from build123d import *

# Parameters (mm, degrees)
SKETCH1_W                = 40
SKETCH1_H                = 30
BOSS_EXTRUDE1_DEPTH      = 15
SKETCH2_W                = 99.5
SKETCH2_H                = 60
BOSS_EXTRUDE2_DEPTH      = 10
M3_CLEARANCE_HOLE1_D     = 3.2
SKETCH7_W                = 105.85
SKETCH7_H                = 66.35
SKETCH7_W_2              = 99.5
SKETCH7_H_2              = 60
BOSS_EXTRUDE3_DEPTH      = 3
CUT_EXTRUDE2_DEPTH       = 1.25
M3_CLEARANCE_HOLE3_D     = 3.2
M3_CLEARANCE_HOLE3_DEPTH = 12
M3_CLEARANCE_HOLE3_TIP   = 0.96137699
F_1_4_CLEARANCE_HOLE3_D  = 6.5278
SKETCH20_R               = 2.8
SKETCH20_R_2             = 5
CUT_EXTRUDE4_DEPTH       = 21
SKETCH23_W               = 6.48
SKETCH23_H               = 3
BOSS_EXTRUDE5_DEPTH      = 10
SKETCH43_W               = 6
SKETCH43_H               = 3
BOSS_EXTRUDE7_DEPTH      = 18
F_1_4_CLEARANCE_HOLE2_D  = 6.5278
CUT_EXTRUDE9_START       = -22
CUT_EXTRUDE9_DEPTH       = 22
SKETCH45_W               = 45
SKETCH45_H               = 60
CUT_EXTRUDE10_DEPTH      = 5
CUT_EXTRUDE11_DEPTH      = 1.25
M3_CLEARANCE_HOLE5_D     = 3.2
M3_CLEARANCE_HOLE5_DEPTH = 10
M3_CLEARANCE_HOLE5_TIP   = 0.96137699
FILLET3_R                = 2
FILLET4_R                = 1


with BuildPart() as part:
    # Sketch1 → Boss-Extrude1 (new body)
    with BuildSketch(Plane(origin=(0, 0, 0), x_dir=(1, 0, 0), z_dir=(0, 1, 0))):
        Rectangle(SKETCH1_W, SKETCH1_H)
    extrude(amount=-BOSS_EXTRUDE1_DEPTH)

    # Sketch2 → Boss-Extrude2 (add)
    with BuildSketch(Plane.XZ.offset(15)):
        with Locations((25.25, 0)):
            Rectangle(SKETCH2_W, SKETCH2_H)
    extrude(amount=BOSS_EXTRUDE2_DEPTH)

    # M3 Clearance Hole1 (through all)
    with Locations(Plane(origin=(0, 0, 0), x_dir=(1, 0, 0), z_dir=(0, 1, 0))):
        with Locations((-16.5, 11.5), (16.5, 11.5), (-16.5, -11.5), (16.5, -11.5)):
            Hole(M3_CLEARANCE_HOLE1_D / 2)

    # Sketch7 → Boss-Extrude3 (add)
    with BuildSketch(Plane.XZ.offset(25)):
        with Locations((25.25, 0)):
            Rectangle(SKETCH7_W, SKETCH7_H)
        with Locations((25.25, 0)):
            Rectangle(SKETCH7_W_2, SKETCH7_H_2, mode=Mode.SUBTRACT)
    extrude(amount=-BOSS_EXTRUDE3_DEPTH)

    # Sketch14 → Cut-Extrude2 (cut, symmetric)
    with BuildSketch(Plane.ZY.offset(20.5)):
        Polygon((-27.75, -16.91228676), (-27.75, -15), (-22.25, -15), (-22.25, -16.91228676), (-22.25, -20.08771324), (-25, -21.675426481), (-27.75, -20.08771324), align=None)
        Polygon((22.25, -16.91228676), (22.25, -20.08771324), (25, -21.675426481), (27.75, -20.08771324), (27.75, -16.91228676), (27.75, -15), (22.25, -15), align=None)
    extrude(amount=CUT_EXTRUDE2_DEPTH, both=True, mode=Mode.SUBTRACT)

    # M3 Clearance Hole3
    with Locations(Plane.ZY.offset(24.5)):
        with Locations((-25, -18.5), (25, -18.5)):
            Hole(M3_CLEARANCE_HOLE3_D / 2, depth=M3_CLEARANCE_HOLE3_DEPTH)
            with Locations((0, 0, -(M3_CLEARANCE_HOLE3_DEPTH + M3_CLEARANCE_HOLE3_TIP / 2))):  # 118° drill point
                Cone(0, M3_CLEARANCE_HOLE3_D / 2, M3_CLEARANCE_HOLE3_TIP, mode=Mode.SUBTRACT)

    # 1/4 Clearance Hole3 (through all)
    with Locations(Plane(origin=(0, 0, 0), x_dir=(1, 0, 0), z_dir=(0, 1, 0))):
        with Locations((-12, 0)):
            Hole(F_1_4_CLEARANCE_HOLE3_D / 2)

    # Sketch20 → Cut-Extrude4 (cut)
    with BuildSketch(Plane.XZ.offset(25)):
        with Locations(Location((-16.5, 11.5, 0), (0, 0, 270))):
            Circle(SKETCH20_R)
        with Locations(Location((16.5, 11.5, 0), (0, 0, 270))):
            Circle(SKETCH20_R)
        with Locations(Location((16.5, -11.5, 0), (0, 0, 270))):
            Circle(SKETCH20_R)
        with Locations(Location((-16.5, -11.5, 0), (0, 0, 270))):
            Circle(SKETCH20_R)
        with Locations(Location((-12, 0, 0), (0, 0, 270))):
            Circle(SKETCH20_R_2)
    extrude(amount=-CUT_EXTRUDE4_DEPTH, mode=Mode.SUBTRACT)

    # Sketch23 → Boss-Extrude5 (add, symmetric)
    with BuildSketch(Plane.XY):
        with Locations((0, -26.5)):
            Rectangle(SKETCH23_W, SKETCH23_H)
    extrude(amount=BOSS_EXTRUDE5_DEPTH, both=True)

    # Sketch43 → Boss-Extrude7 (add)
    with BuildSketch(Plane(origin=(0, -15, 0), x_dir=(1, 0, 0), z_dir=(0, 1, 0))):
        with Locations((-13, 16.5)):
            Rectangle(SKETCH43_W, SKETCH43_H)
        with Locations((-13, -16.5)):
            Rectangle(SKETCH43_W, SKETCH43_H)
        with Locations((13, 16.5)):
            Rectangle(SKETCH43_W, SKETCH43_H)
        with Locations((13, -16.5)):
            Rectangle(SKETCH43_W, SKETCH43_H)
    extrude(amount=BOSS_EXTRUDE7_DEPTH)

    # 1/4 Clearance Hole2 (through all)
    with Locations(Plane(origin=(0, -15, 0), x_dir=(1, 0, 0), z_dir=(0, 1, 0))):
        with Locations((0, 22.5), (0, -22.5)):
            Hole(F_1_4_CLEARANCE_HOLE2_D / 2)

    # Sketch44 → Cut-Extrude9 (cut)
    with BuildSketch(Plane(origin=(0, 0, 0), x_dir=(1, 0, 0), z_dir=(0, 1, 0)).offset(CUT_EXTRUDE9_START)):
        Polygon((-6, 15), (6, 15), (6, 7.5), (20, 7.5), (20, -7.5), (6, -7.5), (6, -15), (-6, -15), align=None)
    extrude(amount=CUT_EXTRUDE9_DEPTH, mode=Mode.SUBTRACT)

    # Sketch45 → Cut-Extrude10 (cut)
    with BuildSketch(Plane(origin=(0, -15, 0), x_dir=(1, 0, 0), z_dir=(0, 1, 0))):
        with Locations((42.5, 0)):
            Rectangle(SKETCH45_W, SKETCH45_H)
    extrude(amount=-CUT_EXTRUDE10_DEPTH, mode=Mode.SUBTRACT)

    # Sketch46 → Cut-Extrude11 (cut, symmetric)
    with BuildSketch(Plane(origin=(71, 0, 0), x_dir=(0, 0, -1), z_dir=(1, 0, 0))):
        Polygon((-2.75, -16.91228676), (-2.75, -15), (2.75, -15), (2.75, -16.91228676), (2.75, -20.08771324), (0, -21.675426481), (-2.75, -20.08771324), align=None)
    extrude(amount=CUT_EXTRUDE11_DEPTH, both=True, mode=Mode.SUBTRACT)

    # M3 Clearance Hole5
    with Locations(Plane(origin=(75, 0, 0), x_dir=(0, 0, -1), z_dir=(1, 0, 0))):
        with Locations((0, -18.5)):
            Hole(M3_CLEARANCE_HOLE5_D / 2, depth=M3_CLEARANCE_HOLE5_DEPTH)
            with Locations((0, 0, -(M3_CLEARANCE_HOLE5_DEPTH + M3_CLEARANCE_HOLE5_TIP / 2))):  # 118° drill point
                Cone(0, M3_CLEARANCE_HOLE5_D / 2, M3_CLEARANCE_HOLE5_TIP, mode=Mode.SUBTRACT)

    # Fillet3
    fillet3_edges = [part.edges().sort_by_distance(p)[0] for p in [
        (-10, -6, -18),
        (-16, -6, -18),
        (-10, -6, 18),
        (-16, -6, 18),
        (10, -6, 18),
        (16, -6, 18),
        (10, -6, -18),
        (16, -6, -18),
        (6, -7.5, 15),
        (6, -11, 7.5),
        (20, -10, 7.5),
        (20, -10, -7.5),
        (6, -11, -7.5),
        (6, -7.5, -15),
        (-6, -7.5, -15),
        (-6, -7.5, 15),
        (20, -17.5, 30),
        (65, -17.5, 30),
        (65, -17.5, -30),
        (20, -17.5, -30),
        (-24.5, -18.5, 30),
        (75, -18.5, 30),
        (75, -18.5, -30),
        (-24.5, -18.5, -30),
        (20, -7.5, 15),
        (-20, -7.5, 15),
        (-20, -7.5, -15),
        (20, -7.5, -15),
    ]]
    fillet(fillet3_edges, radius=FILLET3_R)

    # Fillet4
    fillet4_edges = [part.edges().sort_by_distance(p)[0] for p in [
        (-27.675, -23.5, 33.175),
        (78.175, -23.5, 33.175),
        (78.175, -23.5, -33.175),
        (-27.675, -23.5, -33.175),
    ]]
    fillet(fillet4_edges, radius=FILLET4_R)


solid = part.part
Design review of the part built by this model. Coordinates are the model's own, in mm. A direction names the side the tool comes from. Give positions to 0.01 mm unless a question says otherwise; leave off trailing zeros. Loops run counter-clockwise (first coordinate to the right, second up) from the corner with the lowest first, then second, coordinate; pieces in that order, holes last. Notation, with made-up numbers: (32, 11) - (41, 11) arc R33 cw to (41, 50) - close; hole circle Ø9 at (86, 34.5). An arc over 180 degrees is marked (long way). Use CSV: the item, a comma, the result in double quotes. Start each with the question number.
1. Add section A-A (z = -11.5). Count the separate pieces of the cut face and the enclosed holes in it, plus the area to 3 significant figures.
2. Add section C-C (x = 28.5). State the section outline as (y, z) points (3 decimals).
3. Wall thickness on L1, parallel to X at y = -8.5, z = 11.5; L2, parallel to Z at x = -16.5, y = -1.7; L3, parallel to X at y = -2.35, z = -11.5: over which ranges is each line inside the solid? List them lowest first.
4. Draft analysis for pull direction Y (two halves, no side actions). For faces 1 (the flat face through (-20.482, -20.87, -23.606)), 2 (the flat face through (-20, -7, 0)), 3 (the conical face through (-11.71, -18.22, 24.96)), state which applies: released by +Y, released by -Y, zero draft, split by the parting line, or undercut.
5. Machinability: for faces 4 (the cylindrical face through (-8, -15, -3)), 5 (the flat face through (17, -7, -15)), 6 (the flat face through (-13, -6, 18)), which of the approach directions +Z, -Z, +X, -X, +Y, -Y give a long, thin tool a straight path to every point of the face, cutting with its end or side? Answer none if there is none.
6. Add section B-B (x = 0). State the section outline as (y, z) points (3 decimals), plus the area to 3 significant figures.
7. Insertion check: P1, Ø4.5, axis at y = -9.5, z = -5.5, coming from the -X side; P2, Ø7.5, axis at x = -12, z = 0, coming from the +Y side; P3, Ø4.5, axis at x = 16.5, z = 11.5, coming from the -Y side. Each pin has a flat end and moves straight along its axis. Give the tip position at first contact, or say it passes through.
Results found:
1,separate pieces,"3"
1,enclosed holes,"0"
1,area,"864 mm²"
2,outline,"(-25, -33.175) - (-22, -33.175) - (-22, -30) - (-20, -30) - (-20, 30) - (-22, 30) - (-22, 33.175) - (-25, 33.175) - close"
3,L1,"x = -20 to -19.3, -13.7 to -6, 6 to 13.7, 19.3 to 20"
3,L2,"z = -15 to -13.1, -9.9 to 9.9, 13.1 to 15"
3,L3,"x = -20 to -18.1, -14.9 to -6, 6 to 14.9, 18.1 to 20"
4,face 1,"released by +Y"
4,face 2,"zero draft"
4,face 3,"undercut"
5,face 4,"-Y"
5,face 5,"-Z, +X, +Y"
5,face 6,"+Z, +X, -X, +Y"
6,outline,"(-28, -10) - (-25, -10) - (-25, -19.236) - (-15, -19.236) - (-15, -15) - (-22, -15) - (-22, 15) - (-15, 15) - (-15, 19.236) - (-25, 19.236) - (-25, 10) - (-28, 10) - close; (-25, -33.175) - (-22, -33.175) - (-22, -30) - (-15, -30) - (-15, -25.764) - (-25, -25.764) - close; (-25, 25.764) - (-15, 25.764) - (-15, 30) - (-22, 30) - (-22, 33.175) - (-25, 33.175) - close"
6,area,"338 mm²"
7,P1,"stops at x = -20"
7,P2,"stops at y = 0"
7,P3,"stops at y = -4"
